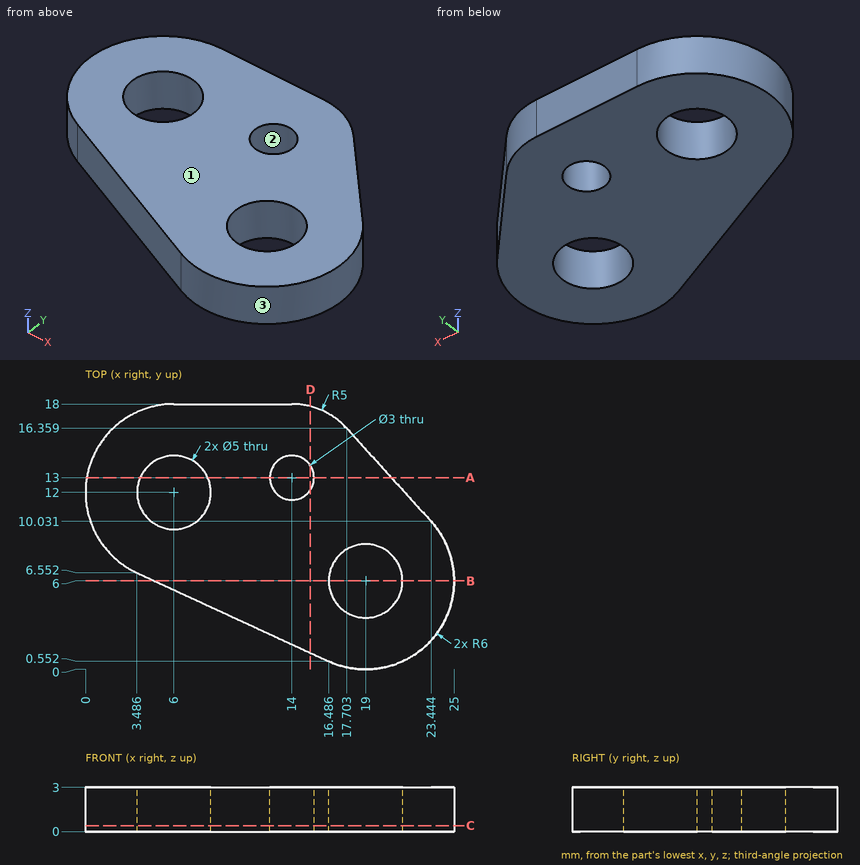
Geometry: see drawing. Coordinates: mm, zero at the bounding-box minimum. Give positions to 0.01 mm unless a question says otherwise; leave off trailing zeros. Loops run counter-clockwise (first coordinate to the right, second up) from the corner with the lowest first, then second, coordinate; pieces in that order, holes last. Notation, with made-up numbers: (52.25, -3) -> (91.25, -3) arc R18 cw to (91.25, 24) -> close; hole circle Ø7 at (87, -8). An arc over 180 degrees is marked (long way). Answer as a JSON object with one key per item and string values. Group by question number.
Item 1: Cut plane A-A, the plane y = 13. Return the cut outline in (x, z).
Item 2: Line query: probe 1 along X at (y, z) = (12, 2.1); probe 2 along X at (y, z) = (14, 1.05) (1 decimal); probe 3 along Y at (x, z) = (20.5, 1.25) (1 decimal). Output: solid intervals per line, ascending.
Item 3: Cut plane D-D, the plane x = 15.25. Return the cut outline in (y, z).
Item 4: Pull-direction query (X, two-part tool) for the marked faces 1, 2 and 3; classes: released by +X, released by -X, zero draft, split by the parting line, or undercut.
Item 5: Cut plane B-B, the plane y = 6. Return the cut outline in (x, z).
Item 6: Cut plane C-C, the plane z = 0.4. Return the cut outline in (x, y) (1 decimal).
Item 7: Pin query (flat end, axial travel): P1, Ø5, axis at x = 20, y = 8, coming from the -Z side; P2, Ø1.5, axis at y = 10, z = 1.5, coming from the +X side. Return the tip coordinate at first contact, or that it passes through.
Checks:
{
 "1": {"outline": "(0.08, 0) -> (3.71, 0) -> (3.71, 3) -> (0.08, 3) -> close; (8.29, 0) -> (12.5, 0) -> (12.5, 3) -> (8.29, 3) -> close; (15.5, 0) -> (20.75, 0) -> (20.75, 3) -> (15.5, 3) -> close"},
 "2": {"probe 1": "x = 0 to 3.5, 8.5 to 12.88, 15.12 to 21.66", "probe 2": "x = 0.3 to 4.5, 7.5 to 12.9, 15.1 to 19.8", "probe 3": "y = 0.2 to 4, 8 to 13.3"},
 "3": {"outline": "(1.12, 0) -> (12.17, 0) -> (12.17, 3) -> (1.12, 3) -> close; (13.83, 0) -> (17.84, 0) -> (17.84, 3) -> (13.83, 3) -> close"},
 "4": {"face 1": "zero draft", "face 2": "undercut", "face 3": "split by the parting line"},
 "5": {"outline": "(4.68, 0) -> (16.5, 0) -> (16.5, 3) -> (4.68, 3) -> close; (21.5, 0) -> (25, 0) -> (25, 3) -> (21.5, 3) -> close"},
 "6": {"outline": "(3.5, 6.6) -> (16.5, 0.6) arc R6 ccw to (23.4, 10) -> (17.7, 16.4) arc R5 ccw to (14, 18) -> (6, 18) arc R6 ccw to start; hole circle Ø5 at (6, 12); hole circle Ø3 at (14, 13); hole circle Ø5 at (19, 6)"},
 "7": {"P1": "stops at z = 0", "P2": "stops at x = 24.04"}
}
